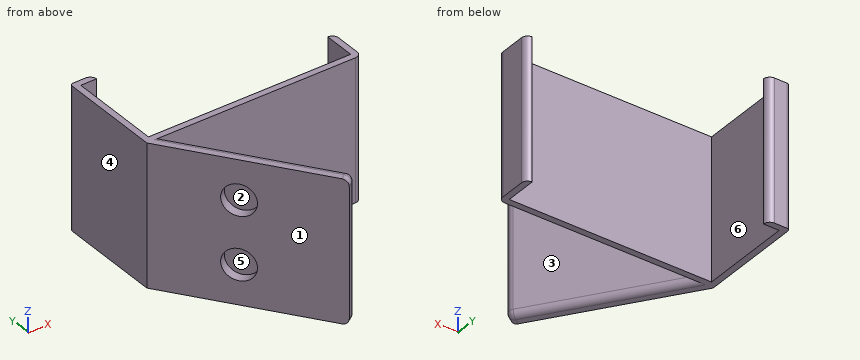
```python
from build123d import *

# Parameters (mm, degrees)
F1_DEPTH = 45
F2_R     = 1.99999
F4_R     = 1
F3_R     = 5
F5_DEPTH = 3.1


# Not quite as in the source:
# - a fillet or chamfer is up to 0.001 mm smaller than in the source, because OpenCascade refuses the exact size
# - a feature names something its author has since deleted; it is built from what else it names


with BuildPart() as f1:
    # F0 (on Top) → F1 (new body)
    with BuildSketch(Plane.XY):
        Polygon((30.2546076554, -42.2925373514), (0, 0), (63.5818746515, 0), (63.5818746515, 12), (61.5818746515, 12), (61.5818746515, 2), (-2.9181253485, 2), (-2.9181253485, 31.5), (2.0818746515, 31.5), (2.0818746515, 33.5), (-4.9181253485, 33.5), (-4.9181253485, 31.5), (-4.9181253485, 0), (27.0013355514, -44.6198148634), align=None)
    extrude(amount=F1_DEPTH)

    # F2 (radius 2 in the source; OpenCascade refuses exactly that, so slightly less here)
    f2_edges = [f1.edges().sort_by_distance(p)[0] for p in [
        (63.581875, 0, 22.5),
        (63.581875, 12, 22.5),
        (30.254608, -42.292537, 22.5),
        (28.627972, -43.456176, 45),
        (28.627972, -43.456176, 0),
        (15.127304, -21.146269, 45),
        (15.127304, -21.146269, 0),
        (2.081875, 33.5, 22.5),
    ]]
    fillet(f2_edges, radius=F2_R)

    # F4
    f4_edges = [f1.edges().sort_by_distance(p)[0] for p in [
        (-4.918125, 33.5, 22.5),
    ]]
    fillet(f4_edges, radius=F4_R)

    # F3 (on face) → F5 (cut)
    with BuildSketch(Plane(origin=(-3.253272104, -2.327277512, 0), x_dir=(0.581819378, -0.813318026, 0), z_dir=(-0.813318026, -0.581819378, 0))):
        with Locations((22.1385393689, 12.5)):
            Circle(F3_R)
        with Locations((22.1385393689, 32.5)):
            Circle(F3_R)
    extrude(amount=-F5_DEPTH, mode=Mode.SUBTRACT)


solid = f1.part
```
Work out the finished part from the listing and answer in its coordinate system (mm). Face numbers are marked on the shaded views. A direction names the side the tool comes from. Coordinates: 2 decimals unless noted, no trailing zeros. Write each loop counter-clockwise with the first axis right and the second up, starting at its lowest first coordinate (ties: lowest second). Pieces come first, ordered by that corner, then holes. Notation, with made-up numbers: (73, -13) - (105, -13) arc R15 ccw to (105, 2) - close; hole circle Ø1 at (-11, 14.25). An arc over 180 degrees is marked (long way). Answer as a JSON object with one key per item and string values.
Q1. Find section D-D (y = 28.5). Write down the section's boundary in (x, z), plus the area to 3 significant figures.
Results list:
{"outline": "(-4.92, 0) - (-2.92, 0) - (-2.92, 45) - (-4.92, 45) - close", "area": "90.0 mm^2"}
Q2. Given pin 1 Ø1.5 at (y, z) = (-20, 15.5) entering from +X; pin 2 Ø6 at (x, z) = (51.5, 5) entering from +Y; pin 3 Ø4 at (x, y) = (51, 2.5) entering from -Z; pin 4 Ø5.5 at (x, z) = (-1, 19.5) entering from -Y, each flat-ended and moving along its own axis, determine where each tip first touches the part or whether it passes through.
Results list:
{"pin 1": "stops at x = 14.84", "pin 2": "stops at y = 2", "pin 3": "stops at z = 0", "pin 4": "stops at y = -9.32"}
Q3. For a pull along X with two mould halves and no side action, classify the marked faces 1, 2 and 3 as pulls with the +X half, pulls with the -X half, needs draft (parallel to the pull), parting line crosses it, or undercut.
Results list:
{"face 1": "pulls with the -X half", "face 2": "undercut", "face 3": "pulls with the +X half"}
Q4. Find section C-C (x = 32). Write down the section's boundary in (y, z), plus the area to 3 significant figures.
Results list:
{"outline": "(0, 0) - (2, 0) - (2, 45) - (0, 45) - close", "area": "90.0 mm^2"}
Q5. Consider L1, parallel to X at y = 10, z = 16; L2, parallel to Y at x = 13, z = 30; L3, parallel to Y at x = 13, z = 10.5. Determine where each line is inside the solid, lowest interval first. Write a range as from..to.
Results list:
{"L1": "x = -4.92..-2.92, 61.58..63.58", "L2": "y = -25.05..-23.24, -19.72..-18.17, 0..2", "L3": "y = -25.05..-23.55, -19.72..-18.17, 0..2"}
Q6. Find section A-A (y = 9). Write down the section's boundary in (x, z), plus the area to 3 significant figures.
Results list:
{"outline": "(-4.92, 0) - (-2.92, 0) - (-2.92, 45) - (-4.92, 45) - close; (61.58, 0) - (63.58, 0) - (63.58, 45) - (61.58, 45) - close", "area": "180 mm^2"}
Q7. Which of the six approach directions +Z, -Z, +X, -X, +Y, -Y give full straight-line access (tool end or side, diameter ignored) to the marked faces 4, 5 and 6?
Results list:
{"face 4": "+Z, -Z, -X, +Y, -Y", "face 5": "none", "face 6": "+Z, -Z"}
